from build123d import *

# Parameters (mm, degrees)
BASE_EXTRUDE_DEPTH           = 50.8
BASE_EXTRUDE_DRAFT           = 3
SKETCH2_W                    = 245.218721479
SKETCH2_H                    = 134.011608982
CUT_EXTRUDE5_DEPTH           = 38.1
CUT_EXTRUDE5_DRAFT           = -5
SKETCH3_R                    = 24.60625
CUT_EXTRUDE1_DEPTH           = 123.388297682
CUT_EXTRUDE1_DRAFT           = -5
CUT_EXTRUDE1_PROFILE_2_DEPTH = 123.388297682
CUT_EXTRUDE1_PROFILE_2_DRAFT = -5
SKETCH5_W                    = 217.80183091
SKETCH5_H                    = 114.879329543
MILL_OUTSIDE_DEPTH           = 123.388297682
SKETCH9_W                    = 228.055799475
SKETCH9_H                    = 112.000717684
MILL_BOSS_DEPTH              = 38.1
SKETCH4_R                    = 25.4
SKETCH4_R_2                  = 6.35
SKETCH4_R_3                  = 4.7625
BORES_AND_HOLES_DEPTH        = 118.359218484
SKETCH18_R                   = 3.175
SET_SCREW_HOLES_DEPTH        = 38.1


with BuildPart() as part:
    # Sketch1 → Base-Extrude (with draft: the straight prism first)
    with BuildSketch(Plane.XY):
        with BuildLine():
            Line((99.7585, -28.575), (99.7585, 28.575))
            ThreePointArc((99.7585, 28.575), (96.113150999, 37.375650999), (87.3125, 41.021))
            Line((87.3125, 41.021), (-87.3125, 41.021))
            ThreePointArc((-87.3125, 41.021), (-96.113150999, 37.375650999), (-99.7585, 28.575))
            Line((-99.7585, 28.575), (-99.7585, -28.575))
            ThreePointArc((-99.7585, -28.575), (-96.113150999, -37.375650999), (-87.3125, -41.021))
            Line((-87.3125, -41.021), (87.3125, -41.021))
            ThreePointArc((87.3125, -41.021), (96.113150999, -37.375650999), (99.7585, -28.575))
        make_face()
    extrude(amount=-BASE_EXTRUDE_DEPTH)
    # Base-Extrude: the draft: its side faces are tilted about the plane it starts from
    base_extrude_sides = [part.faces().sort_by_distance(p)[0] for p in [
        (99.7585, 0, -25.4),
        (96.113150999, 37.375650999, -25.4),
        (0, 41.021, -25.4),
        (-96.113150999, 37.375650999, -25.4),
        (-99.7585, 0, -25.4),
        (-96.113150999, -37.375650999, -25.4),
        (0, -41.021, -25.4),
        (96.113150999, -37.375650999, -25.4),
    ]]
    draft(base_extrude_sides, Plane.XY, BASE_EXTRUDE_DRAFT)


with BuildPart() as cut_extrude5_tool:
    # Sketch2 → Cut-Extrude5 (with draft: the straight prism first)
    with BuildSketch(Plane.XY):
        with Locations((-2.312638736, -3.991522499)):
            Rectangle(SKETCH2_W, SKETCH2_H)
        with BuildLine():
            Line((-21.652420857, 19.05), (21.652420857, 19.05))
            ThreePointArc((21.652420857, 19.05), (26.837174146, 20.156539199), (31.118441962, 23.283333333))
            ThreePointArc((31.118441962, 23.283333333), (92.075, 0), (31.118441962, -23.283333333))
            ThreePointArc((31.118441962, -23.283333333), (26.837174146, -20.156539199), (21.652420857, -19.05))
            Line((21.652420857, -19.05), (-21.652420857, -19.05))
            ThreePointArc((-21.652420857, -19.05), (-26.837174146, -20.156539199), (-31.118441962, -23.283333333))
            ThreePointArc((-31.118441962, -23.283333333), (-92.075, 0), (-31.118441962, 23.283333333))
            ThreePointArc((-31.118441962, 23.283333333), (-26.837174146, 20.156539199), (-21.652420857, 19.05))
        make_face(mode=Mode.SUBTRACT)
    extrude(amount=-CUT_EXTRUDE5_DEPTH)
    # Cut-Extrude5: the draft: its side faces are tilted about the plane it starts from
    cut_extrude5_sides = [cut_extrude5_tool.faces().sort_by_distance(p)[0] for p in [
        (-124.921999475, -3.991522499, -19.05),
        (-2.312638735, -70.99732699, -19.05),
        (120.296722004, -3.991522499, -19.05),
        (-2.312638735, 63.014281992, -19.05),
        (-26.837174146, 20.156539199, -19.05),
        (0, 19.05, -19.05),
        (26.837174146, 20.156539199, -19.05),
        (92.075, 0, -19.05),
        (26.837174146, -20.156539199, -19.05),
        (0, -19.05, -19.05),
        (-26.837174146, -20.156539199, -19.05),
        (-92.075, 0, -19.05),
    ]]
    draft(cut_extrude5_sides, Plane.XY, CUT_EXTRUDE5_DRAFT)


with BuildPart() as part_1:
    add(part.part)

    # Cut-Extrude5: cut by cut_extrude5_tool
    add(cut_extrude5_tool.part, mode=Mode.SUBTRACT)


with BuildPart() as cut_extrude1_tool:
    # Sketch3 → Cut-Extrude1 (with draft: the straight prism first)
    with BuildSketch(Plane(origin=(0, 0, -50.8), x_dir=(-1, 0, 0), z_dir=(0, 0, -1))):
        with Locations((57.15, 0)):
            Circle(SKETCH3_R)
    extrude(amount=-CUT_EXTRUDE1_DEPTH)
    # Cut-Extrude1: the draft: its side faces are tilted about the plane it starts from
    cut_extrude1_sides = [cut_extrude1_tool.faces().sort_by_distance(p)[0] for p in [
        (-32.54375, 0, 10.894148841),
    ]]
    draft(cut_extrude1_sides, Plane(origin=(0, 0, -50.8), x_dir=(-1, 0, 0), z_dir=(0, 0, -1)), CUT_EXTRUDE1_DRAFT)


with BuildPart() as part_2:
    add(part_1.part)

    # Cut-Extrude1: cut by cut_extrude1_tool
    add(cut_extrude1_tool.part, mode=Mode.SUBTRACT)


with BuildPart() as cut_extrude1_profile_2_tool:
    # Sketch3 → Cut-Extrude1 profile 2 (with draft: the straight prism first)
    with BuildSketch(Plane(origin=(0, 0, -50.8), x_dir=(-1, 0, 0), z_dir=(0, 0, -1))):
        with Locations((-57.15, 0)):
            Circle(SKETCH3_R)
    extrude(amount=-CUT_EXTRUDE1_PROFILE_2_DEPTH)
    # Cut-Extrude1 profile 2: the draft: its side faces are tilted about the plane it starts from
    cut_extrude1_profile_2_sides = [cut_extrude1_profile_2_tool.faces().sort_by_distance(p)[0] for p in [
        (81.75625, 0, 10.894148841),
    ]]
    draft(cut_extrude1_profile_2_sides, Plane(origin=(0, 0, -50.8), x_dir=(-1, 0, 0), z_dir=(0, 0, -1)), CUT_EXTRUDE1_PROFILE_2_DRAFT)


with BuildPart() as part_3:
    add(part_2.part)

    # Cut-Extrude1 profile 2: cut by cut_extrude1_profile_2_tool
    add(cut_extrude1_profile_2_tool.part, mode=Mode.SUBTRACT)

    # Sketch5 → Mill outside (cut, through all)
    with BuildSketch(Plane.XY):
        with Locations((-0.351671417, -5.861190283)):
            Rectangle(SKETCH5_W, SKETCH5_H)
        with BuildLine():
            Line((98.171, -28.575), (98.171, 28.575))
            ThreePointArc((98.171, 28.575), (94.990618984, 36.253118984), (87.3125, 39.4335))
            Line((87.3125, 39.4335), (-87.3125, 39.4335))
            ThreePointArc((-87.3125, 39.4335), (-94.990618984, 36.253118984), (-98.171, 28.575))
            Line((-98.171, 28.575), (-98.171, -28.575))
            ThreePointArc((-98.171, -28.575), (-94.990618984, -36.253118984), (-87.3125, -39.4335))
            Line((-87.3125, -39.4335), (87.3125, -39.4335))
            ThreePointArc((87.3125, -39.4335), (94.990618984, -36.253118984), (98.171, -28.575))
        make_face(mode=Mode.SUBTRACT)
    extrude(amount=-MILL_OUTSIDE_DEPTH, mode=Mode.SUBTRACT)

    # Sketch9 → Mill boss (cut)
    with BuildSketch(Plane.XY):
        with Locations((8.711546203, 4.265795104)):
            Rectangle(SKETCH9_W, SKETCH9_H)
        with BuildLine():
            Line((-21.652420857, -15.0876), (21.652420857, -15.0876))
            ThreePointArc((21.652420857, -15.0876), (28.454817172, -16.53937943), (34.071840547, -20.641733333))
            ThreePointArc((34.071840547, -20.641733333), (88.1126, 0), (34.071840547, 20.641733333))
            ThreePointArc((34.071840547, 20.641733333), (28.454817172, 16.53937943), (21.652420857, 15.0876))
            Line((21.652420857, 15.0876), (-21.652420857, 15.0876))
            ThreePointArc((-21.652420857, 15.0876), (-28.454817172, 16.53937943), (-34.071840547, 20.641733333))
            ThreePointArc((-34.071840547, 20.641733333), (-88.1126, 0), (-34.071840547, -20.641733333))
            ThreePointArc((-34.071840547, -20.641733333), (-28.454817172, -16.53937943), (-21.652420857, -15.0876))
        make_face(mode=Mode.SUBTRACT)
    extrude(amount=-MILL_BOSS_DEPTH, mode=Mode.SUBTRACT)

    # Sketch4 → Bores and holes (cut, through all)
    with BuildSketch(Plane(origin=(0, 0, -50.8), x_dir=(-1, 0, 0), z_dir=(0, 0, -1))):
        with Locations((-57.15, 0)):
            Circle(SKETCH4_R)
        with Locations((57.15, 0)):
            Circle(SKETCH4_R)
        Circle(SKETCH4_R_2)
        with Locations((-87.3252, 28.575)):
            Circle(SKETCH4_R_3)
        with Locations((-87.3252, -28.575)):
            Circle(SKETCH4_R_3)
        with Locations((87.2998, -28.575)):
            Circle(SKETCH4_R_3)
        with Locations((87.2998, 28.575)):
            Circle(SKETCH4_R_3)
    extrude(amount=-BORES_AND_HOLES_DEPTH, mode=Mode.SUBTRACT)

    # Sketch18 → Set screw holes (cut)
    with BuildSketch(Plane(origin=(0, 0, 0), x_dir=(1, 0, 0), z_dir=(0, 1, 0))):
        with Locations(Location((0, 6.35, 0), (0, 0, 90))):
            Circle(SKETCH18_R)
        with Locations(Location((0, 31.75, 0), (0, 0, 90))):
            Circle(SKETCH18_R)
    extrude(amount=SET_SCREW_HOLES_DEPTH, mode=Mode.SUBTRACT)


solid = part_3.part
Design review of the part built by this model. Coordinates are the model's own, in mm. A direction names the side the tool comes from. Give positions to 0.01 mm unless a question says otherwise; leave off trailing zeros. Loops run counter-clockwise (first coordinate to the right, second up) from the corner with the lowest first, then second, coordinate; pieces in that order, holes last. Notation, with made-up numbers: (-10.5, 81.5) - (26.5, 81.5) arc R18 ccw to (26.5, 109.5) - close; hole circle Ø9 at (73.5, 0). An arc over 180 degrees is marked (long way). Write item = value, one per line.
1) Take a section at A-A on x = 0. Count the separate pieces of the cut face and the enclosed holes in it, and give its area (3 significant figures).
Result sheet:
separate_pieces = 4
enclosed_holes = 0
area = 1,400 mm2
2) Take a section at D-D on y = 13. State the section outline as (x, z) points (3 decimals).
Result sheet:
outline = (-98.171, -50.8) - (-78.971, -50.8) - (-78.971, 0) - (-85.251, 0) - (-85.251, -38.1) - (-98.171, -38.1) - close; (-35.329, -50.8) - (35.329, -50.8) - (35.329, 0) - (-35.329, 0) - close; (78.971, -50.8) - (98.171, -50.8) - (98.171, -38.1) - (85.251, -38.1) - (85.251, 0) - (78.971, 0) - close; hole circle Ø6.35 at (0, -31.75); hole circle Ø6.35 at (0, -6.35)
3) Tool access review of faces 5 (the face through (-1, 18, -38.1)), 6 (the face through (28.544, 16.58, -18.783)), 7 (the face through (-0.95, 10.23, -9.38)): name each direction out of +Z, -Z, +X, -X, +Y, -Y from which nothing blocks a thin tool from reaching the whole face with its end or side.
Result sheet:
face_5 = +Z
face_6 = +Z, +Y
face_7 = +Y
4) Draft analysis for pull direction X (two halves, no side actions). For faces 1 (the face through (-28.37, 16.5, -18.78)), 2 (the face through (94.906, -36.337, -44.361)), 3 (the face through (-89.86, -24.56, -44.54)), 4 (the face through (-1, 9, -50.8)), state which applies: +X half, -X half, draft (parallel to the pull), parting line (faces both ways), or undercut.
Result sheet:
face_1 = undercut
face_2 = +X half
face_3 = undercut
face_4 = draft
5) Take a section at B-B on z = -15.5. State the section outline as (x, y) points, and give its area (3 significant figures).
Result sheet:
outline = (-34.07, -20.64) arc R16.66 cw to (-21.65, -15.09) - (21.65, -15.09) arc R16.66 cw to (34.07, -20.64) arc R30.96 ccw (long way) to (34.07, 20.64) arc R16.66 cw to (21.65, 15.09) - (-21.65, 15.09) arc R16.66 cw to (-34.07, 20.64) arc R30.96 ccw (long way) to start; hole circle Ø50.8 at (-57.15, 0); hole circle Ø12.7 at (0, 0); hole circle Ø50.8 at (57.15, 0)
area = 3,540 mm2
6) Take a section at C-C on x = -57.15. State the section outline as (y, z) points.
Result sheet:
outline = (-39.43, -50.8) - (-25.4, -50.8) - (-25.4, 0) - (-30.96, 0) - (-30.96, -38.1) - (-39.43, -38.1) - close; (25.4, -50.8) - (39.43, -50.8) - (39.43, -38.1) - (30.96, -38.1) - (30.96, 0) - (25.4, 0) - close
7) To check wall thickness, follow line 1 (X direction, y = -5, z = -46.5); line 2 (X direction, y = 20, z = -37); line 3 (Y direction, x = -85, z = -38.5). State the ranges of each line that lie inside material, in increasing order.
Result sheet:
line_1 = -98.17 to -82.05, -32.25 to -3.91, 3.91 to 32.25, 82.05 to 98.17
line_2 = -80.79 to -72.81, -41.49 to -33.47, 33.47 to 41.49, 72.81 to 80.79
line_3 = -39.43 to -32.75, -24.4 to 24.4, 32.75 to 39.43
8) Clearance check with flat-ended pins moving along their axes: pin 1 Ø4 at (x, z) = (0, -31.75) entering from +Y; pin 2 Ø19 at (x, z) = (1, -18.5) entering from +Y; pin 3 Ø10 at (x, z) = (41.5, -18.5) entering from +Y. State where each tip first meets the part, or that it passes through.
Result sheet:
pin_1 = -6.03
pin_2 = 15.09
pin_3 = 29.07
